```python
from build123d import *

# Parameters (mm, degrees)
EXTRUDE_1_DEPTH     = 10
SKETCH_2_W          = 10
SKETCH_2_H          = 18
EXTRUDE_2_DEPTH     = 3
SKETCH_3_R          = 1.2
CUT_EXTRUDE_1_DEPTH = 99.701570403
SKETCH_4_W          = 150
SKETCH_4_H          = 2
EXTRUDE_3_DEPTH     = 2
SKETCH_5_W          = 19
SKETCH_5_H          = 34.5
EXTRUDE_4_DEPTH     = 3.1
SKETCH_7_W          = 8
SKETCH_7_H          = 2.3
CUT_EXTRUDE_2_DEPTH = 10
FILLET_1_R          = 1


with BuildPart() as part:
    # Эскиз1 → Бобышка-Вытянуть1 (new body)
    with BuildSketch(Plane(origin=(0, 0, 0), x_dir=(1, 0, 0), z_dir=(0, 1, 0))):
        Polygon((-87, 21.5), (-87, 18.5), (-60, 18.5), (60, 18.5), (60, -21.5), (63, -21.5), (63, 21.5), align=None)
    extrude(amount=EXTRUDE_1_DEPTH)

    # Эскиз2 → Бобышка-Вытянуть2 (add)
    with BuildSketch(Plane(origin=(0, 0, -21.5), x_dir=(-1, 0, 0), z_dir=(0, 0, -1))):
        with Locations((52, 9)):
            Rectangle(SKETCH_2_W, SKETCH_2_H)
    extrude(amount=-EXTRUDE_2_DEPTH)

    # Эскиз3 → Вырез-Вытянуть1 (cut, through all)
    with BuildSketch(Plane(origin=(0, 0, -21.5), x_dir=(-1, 0, 0), z_dir=(0, 0, -1))):
        with Locations((52, 15)):
            Circle(SKETCH_3_R)
        with Locations((52, 5)):
            Circle(SKETCH_3_R)
    extrude(amount=-CUT_EXTRUDE_1_DEPTH, mode=Mode.SUBTRACT)

    # Эскиз4 → Бобышка-Вытянуть3 (add)
    with BuildSketch(Plane(origin=(0, 0, -21.5), x_dir=(-1, 0, 0), z_dir=(0, 0, -1))):
        with Locations((12, 1)):
            Rectangle(SKETCH_4_W, SKETCH_4_H)
    extrude(amount=EXTRUDE_3_DEPTH)

    # Эскиз5 → Бобышка-Вытянуть4 (add)
    with BuildSketch(Plane.XY.offset(-18.5)):
        with Locations((-77.5, 17.25)):
            Rectangle(SKETCH_5_W, SKETCH_5_H)
    extrude(amount=-EXTRUDE_4_DEPTH)

    # Эскиз7 → Вырез-Вытянуть2 (cut)
    with BuildSketch(Plane.XY.offset(-18.5)):
        with Locations((-73.5, 30.850007469)):
            Rectangle(SKETCH_7_W, SKETCH_7_H)
        with Locations((-81.5, 5.639796257)):
            Rectangle(SKETCH_7_W, SKETCH_7_H)
    extrude(amount=-CUT_EXTRUDE_2_DEPTH, mode=Mode.SUBTRACT)

    # Скругление1
    fillet_1_edges = [part.edges().sort_by_distance(p)[0] for p in [
        (-85.5, 4.489796257, -20.05),
        (-85.5, 6.789796257, -20.05),
        (-77.5, 6.789796257, -20.05),
        (-77.5, 4.489796257, -20.05),
        (-69.5, 32.000007469, -20.05),
        (-69.5, 29.700007469, -20.05),
        (-77.5, 29.700007469, -20.05),
        (-77.5, 32.000007469, -20.05),
    ]]
    fillet(fillet_1_edges, radius=FILLET_1_R)


solid = part.part
```
Read the model definition and answer for the solid it produces. Units are mm, in the model's axes. A direction names the side the tool comes from. Coordinates: 2 decimals unless noted, no trailing zeros. Order: outer loops, then holes, each group sorted by start corner. A loop starts at its lowest first (then second) coordinate and runs counter-clockwise, first axis right, second up. Notation, with made-up numbers: (56.25, -15.75) - (66.25, -15.75) arc R4 cw to (66.25, -9.75) - close; hole circle Ø2 at (-38, -2). An arc over 180 degrees is marked (long way). Answer as a JSON object with one key per item and string values. Group by question number.
Item 1: The mould has two halves that part along Y. Classify faces 6 (the face through (-78, 18, -21.6)), 7 (the face through (-52, 18, -20)), 8 (the face through (-82, 4.49, -20)), 9 (the face through (-82, 6.79, -20)): +Y half, -Y half, draft (parallel to the pull), parting line (faces both ways), or undercut.
Item 2: Consider probe 1 along Y at (x, z) = (-52, -19.45); probe 2 along Z at (x, y) = (-72.5, 22.5); probe 3 along Z at (x, y) = (-61, 5.5). Determine where each line is inside the solid, lowest interval first. Write a range as from..to.
Item 3: Section A-A (x = 17) is taken. Give the vertices of the cut face in (y, z), plus the area to 3 significant figures.
Item 4: Section B-B (z = 9.5) is taken. Give the vertices of the cut face in (x, y).
Item 5: A tool of negligible diameter and unlimited length cuts with its end or side. For faces 1 (the face through (24, 10, -19)), 2 (the face through (60, 5, 1)), 3 (the face through (-2, 6, -21.5)), 4 (the face through (-74, 29.7, -20)), 5 (the face through (-63, 10, -20)), from which of +Z, -Z, +X, -X, +Y, -Y can it reach the whole face along a straight path? Write none if from no direction.
Item 6: Section C-C (y = 27) is taken. Give the vertices of the cut face in (x, z).
Item 7: Flat-ended cylindrical pins translate along their axes: P1, Ø5.5, axis at x = -79, y = 22.5, coming from the -Z side; P2, Ø1, axis at x = -13, y = 10, coming from the +Z side; P3, Ø3, axis at y = 5, z = -2, coming from the -X side. Find the tip coordinate at first contact, or state that the pin passes through.
Results are:
{
 "1": {"face 6": "draft", "face 7": "+Y half", "face 8": "undercut", "face 9": "undercut"},
 "2": {"probe 1": "y = 0..3.8, 6.2..13.8, 16.2..18", "probe 2": "z = -21.6..-18.5", "probe 3": "z = -21.5..-18.5"},
 "3": {"outline": "(0, -23.5) - (2, -23.5) - (2, -21.5) - (10, -21.5) - (10, -18.5) - (0, -18.5) - close", "area": "34.0 mm^2"},
 "4": {"outline": "(60, 0) - (63, 0) - (63, 10) - (60, 10) - close"},
 "5": {"face 1": "+Z, -Z, +X, +Y", "face 2": "+Z, -X, +Y, -Y", "face 3": "-Z, +X, +Y", "face 4": "+Z, -Z", "face 5": "+Z, -Z, +Y"},
 "6": {"outline": "(-87, -21.6) - (-68, -21.6) - (-68, -18.5) - (-87, -18.5) - close"},
 "7": {"P1": "stops at z = -21.6", "P2": "stops at z = -18.5", "P3": "stops at x = 60"}
}
